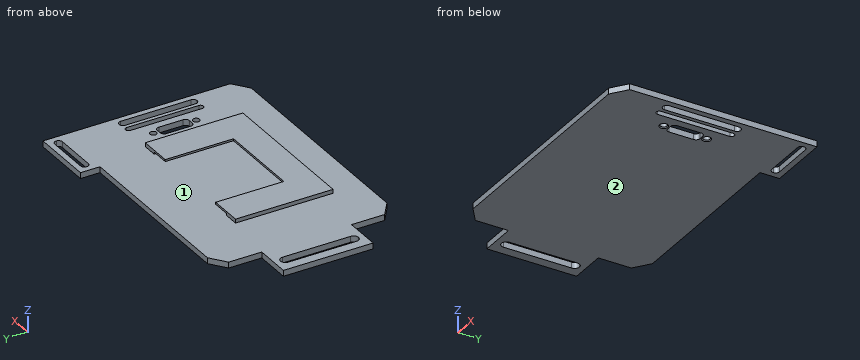
```python
from build123d import *

# Parameters (mm, degrees)
SKETCH029_W     = 62
SKETCH029_H     = 40
PAD002_DEPTH    = 2
SKETCH030_W     = 40
SKETCH030_H     = 1
POCKET001_DEPTH = 9.5
SKETCH031_W     = 40
SKETCH031_H     = 1
POCKET002_DEPTH = 9.5
SKETCH032_W     = 43
SKETCH032_H     = 1
POCKET003_DEPTH = 5
PAD_DEPTH       = 3
SKETCH027_R     = 1.7
SKETCH027_W     = 6.5
SKETCH027_H     = 16.5
SKETCH027_W_2   = 4
SKETCH027_H_2   = 40
SKETCH027_W_3   = 3
SKETCH027_W_4   = 26
SKETCH027_H_3   = 4
SKETCH027_W_5   = 5
POCKET_DEPTH    = 3
FILLET001_R     = 1.9999
FILLET002_R     = 1.4999
FILLET003_R     = 2.4999
CHAMFER001_SIZE = 0.5
SKETCH028_W     = 77
SKETCH028_H     = 50
PAD001_DEPTH    = 2


with BuildPart() as body002:
    # Sketch029 → Pad002 (new body)
    with BuildSketch(Plane.XY):
        Rectangle(SKETCH029_W, SKETCH029_H)
    extrude(amount=PAD002_DEPTH)

    # Sketch030 (on Face2 of Pad002) → Pocket001 (cut)
    with BuildSketch(Plane.YZ.offset(31)):
        with Locations((0, 1.5)):
            Rectangle(SKETCH030_W, SKETCH030_H)
    extrude(amount=-POCKET001_DEPTH, mode=Mode.SUBTRACT)

    # Sketch031 (on Face7 of Pocket001) → Pocket002 (cut)
    with BuildSketch(Plane(origin=(-31, 0, 0), x_dir=(0, -1, 0), z_dir=(-1, 0, 0))):
        with Locations((0, 1.5)):
            Rectangle(SKETCH031_W, SKETCH031_H)
    extrude(amount=-POCKET002_DEPTH, mode=Mode.SUBTRACT)

    # Sketch032 (on Face10 of Pocket002) → Pocket003 (cut)
    with BuildSketch(Plane.XZ.offset(20)):
        with Locations((0, 1.5)):
            Rectangle(SKETCH032_W, SKETCH032_H)
    extrude(amount=-POCKET003_DEPTH, mode=Mode.SUBTRACT)


with BuildPart() as body002_1:
    # Body002 placement: moved
    add(body002.part.moved(Location((0, 0, 3))))


with BuildPart() as chest_mount:
    # Sketch → Pad (new body)
    with BuildSketch(Plane.XY):
        Polygon((-57.9, 46), (33.9, 46), (33.9, 56), (65.9, 56), (65.9, -40), (57.9, -46), (-57.9, -46), (-65.9, -40), (-65.9, -23), (-84.4, -23), (-84.4, 23), (-65.9, 23), (-65.9, 40), align=None)
    extrude(amount=PAD_DEPTH)

    # Sketch027 (on Face15 of Pad) → Pocket (cut)
    with BuildSketch(Plane.XY.offset(3)):
        with Locations((46.65, 11)):
            Circle(SKETCH027_R)
        with Locations((46.65, -11)):
            Circle(SKETCH027_R)
        with Locations((46.65, 0)):
            Rectangle(SKETCH027_W, SKETCH027_H)
        with Locations((60.9, 0)):
            Rectangle(SKETCH027_W_2, SKETCH027_H_2)
        with Locations((55.4, 0)):
            Rectangle(SKETCH027_W_3, SKETCH027_H_2)
        with Locations((49.9, 51)):
            Rectangle(SKETCH027_W_4, SKETCH027_H_3)
        with Locations((-76.9, 0)):
            Rectangle(SKETCH027_W_5, SKETCH027_H_2)
    extrude(amount=-POCKET_DEPTH, mode=Mode.SUBTRACT)

    # Fillet001
    fillet001_edges = [chest_mount.edges().sort_by_distance(p)[0] for p in [
        (62.9, 20, 1.5),
        (58.9, 20, 1.5),
        (62.9, -20, 1.5),
        (58.9, -20, 1.5),
        (36.9, 49, 1.5),
        (62.9, 49, 1.5),
        (62.9, 53, 1.5),
        (36.9, 53, 1.5),
        (49.9, -8.25, 1.5),
        (43.4, -8.25, 1.5),
        (43.4, 8.25, 1.5),
        (49.9, 8.25, 1.5),
    ]]
    fillet(fillet001_edges, radius=FILLET001_R)

    # Fillet002
    fillet002_edges = [chest_mount.edges().sort_by_distance(p)[0] for p in [
        (53.9, -20, 1.5),
        (56.9, -20, 1.5),
        (53.9, 20, 1.5),
        (56.9, 20, 1.5),
    ]]
    fillet(fillet002_edges, radius=FILLET002_R)

    # Fillet003
    fillet003_edges = [chest_mount.edges().sort_by_distance(p)[0] for p in [
        (-74.4, -20, 1.5),
        (-79.4, -20, 1.5),
        (-79.4, 20, 1.5),
        (-74.4, 20, 1.5),
    ]]
    fillet(fillet003_edges, radius=FILLET003_R)

    # Chamfer001
    chamfer001_edges = [chest_mount.edges().sort_by_distance(p)[0] for p in [
        (44.95, 11, 0),
        (44.95, -11, 0),
    ]]
    chamfer(chamfer001_edges, length=CHAMFER001_SIZE)

    # Sketch028 (on Face58 of Chamfer001) → Pad001 (join)
    with BuildSketch(Plane.XY.offset(3)):
        with Locations((0, -5)):
            Rectangle(SKETCH028_W, SKETCH028_H)
    extrude(amount=PAD001_DEPTH)

    # Boolean: cut Body002
    add(body002_1.part, mode=Mode.SUBTRACT)


solid = chest_mount.part
```
For this review, take the finished solid that the model builds, in its own axes (mm). Face numbers are marked on the shaded views. Round coordinates to 2 decimals unless told otherwise and drop trailing zeros. Write each loop counter-clockwise with the first axis right and the second up, starting at its lowest first coordinate (ties: lowest second). Pieces come first, ordered by that corner, then holes. Notation, with made-up numbers: (61, -23.5) - (120, -23.5) arc R25 ccw to (120, 12.5) - close; hole circle Ø8 at (23.5, -4.75). An arc over 180 degrees is marked (long way). Write each question's results on one line, items separated by ' | '.
Item 1: Take a section at B-B on x = 4.5. State the section outline as (y, z) points.
Calculated:
outline: (-46, 0) - (46, 0) - (46, 3) - (-20, 3) - (-20, 4) - (-15, 4) - (-15, 5) - (-30, 5) - (-30, 3) - (-46, 3) - close
Item 2: Take a section at A-A on y = -2. Count the separate pieces of the cut face and the enclosed holes in it, then the cut area to 3 significant figures.
Calculated:
separate pieces: 5 | enclosed holes: 0 | area: 444 mm^2
Item 3: To check wall thickness, follow line 1 along Y through (x, z) = (46.65, 2.1); line 2 along Y through (x, z) = (42, 2.2); line 3 along X through (y, z) = (15, 4.6). State the ranges of each line that lie inside material, in increasing order. Write a range as from..to.
Calculated:
line 1: y = -46..-12.7, -9.3..-8.25, 8.25..9.3, 12.7..49, 53..56 | line 2: y = -46..49, 53..56 | line 3: x = -38.5..-21.5, 21.5..38.5
Item 4: For pin 1 (0.6 mm diameter, centred on x = -26, z = 3.5, fed in from +Y); pin 2 (8 mm diameter, centred on x = 35.5, y = 35.5, fed in from +Z); pin 3 (0.5 mm diameter, centred on y = 2.5, z = 4.5, fed in from +X), all flat-tipped, find the tip position at first contact; note any pin that passes through.
Calculated:
pin 1: stops at y = -20 | pin 2: stops at z = 3 | pin 3: stops at x = 38.5
Item 5: Draft analysis for pull direction X (two halves, no side actions). For the marked faces 1 and 2, state which applies: pulls with the +X half, pulls with the -X half, needs draft (parallel to the pull), parting line crosses it, or undercut.
Calculated:
face 1: undercut | face 2: needs draft
Item 6: Take a section at D-D on x = -32.5. State the section outline as (y, z) points, then the cut area to 3 significant figures.
Calculated:
outline: (-46, 0) - (46, 0) - (46, 3) - (20, 3) - (20, 5) - (-30, 5) - (-30, 3) - (-46, 3) - close | area: 376 mm^2
